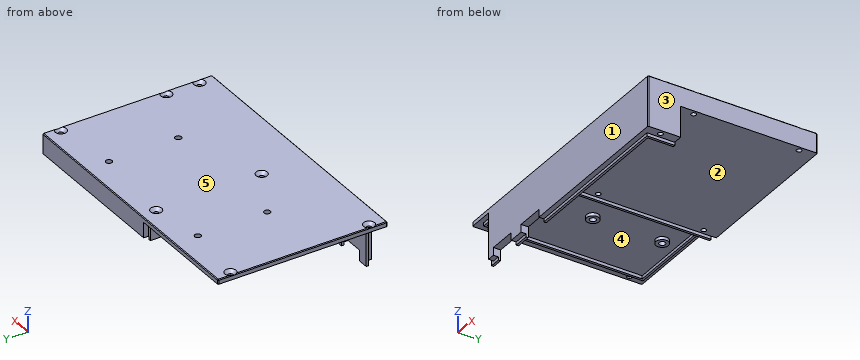
from build123d import *

# Parameters (mm, degrees)
ESQUISSE1_W             = 177.7
ESQUISSE1_H             = 110
BOSS_EXTRU_1_DEPTH      = 3
ESQUISSE2_W             = 102.6
ESQUISSE2_H             = 88.6
BOSS_EXTRU_2_DEPTH      = 10
BOSS_EXTRU_3_DEPTH      = 30
ESQUISSE4_W             = 6.1
ESQUISSE4_H             = 20
ENL_V_MAT_EXTRU_1_DEPTH = 0.2
ESQUISSE5_W             = 10
ESQUISSE5_H             = 3.2
ENL_V_MAT_EXTRU_2_DEPTH = 0.2
BOSS_EXTRU_4_DEPTH      = 2
BOSS_EXTRU_5_DEPTH      = 10
BOSS_EXTRU_6_DEPTH      = 30
ESQUISSE9_R             = 1.6
ENL_V_MAT_EXTRU_3_DEPTH = 212.901604524
CHANFREIN1_SIZE         = 2
CHANFREIN2_SIZE         = 0.5
ESQUISSE10_R            = 2
ENL_V_MAT_EXTRU_4_DEPTH = 5
ESQUISSE11_R            = 4
ESQUISSE11_R_2          = 2
BOSS_EXTRU_7_DEPTH      = 5
ESQUISSE13_W            = 18
ESQUISSE13_H            = 4.7
ENL_V_MAT_EXTRU_5_DEPTH = 7
ESQUISSE14_W            = 96.5
ESQUISSE14_H            = 0.5
BOSS_EXTRU_8_DEPTH      = 2


with BuildPart() as part:
    # Esquisse1 → Boss.-Extru.1 (new body)
    with BuildSketch(Plane.XY):
        with Locations((88.85, 55)):
            Rectangle(ESQUISSE1_W, ESQUISSE1_H)
    extrude(amount=BOSS_EXTRU_1_DEPTH)

    # Esquisse2 → Boss.-Extru.2 (add)
    with BuildSketch(Plane(origin=(0, 0, 0), x_dir=(-1, 0, 0), z_dir=(0, 0, -1))):
        with Locations((-126.4, 65.7)):
            Rectangle(ESQUISSE2_W, ESQUISSE2_H)
    extrude(amount=BOSS_EXTRU_2_DEPTH)

    # Esquisse3 → Boss.-Extru.3 (add)
    with BuildSketch(Plane(origin=(0, 0, 0), x_dir=(-1, 0, 0), z_dir=(0, 0, -1))):
        Polygon((-177.7, 21.4), (-171.6, 21.4), (-171.6, 3.2), (-16.2, 3.2), (-16.2, 0), (-177.7, 0), align=None)
    extrude(amount=BOSS_EXTRU_3_DEPTH)

    # Esquisse4 → Enlèv. mat.-Extru.1 (cut)
    with BuildSketch(Plane(origin=(0, 21.4, 0), x_dir=(1, 0, 0), z_dir=(0, 1, 0))):
        with Locations((174.65, 20)):
            Rectangle(ESQUISSE4_W, ESQUISSE4_H)
    extrude(amount=-ENL_V_MAT_EXTRU_1_DEPTH, mode=Mode.SUBTRACT)

    # Esquisse5 → Enlèv. mat.-Extru.2 (cut)
    with BuildSketch(Plane.ZY.offset(-75.1)):
        with Locations((-5, 108.4)):
            Rectangle(ESQUISSE5_W, ESQUISSE5_H)
    extrude(amount=-ENL_V_MAT_EXTRU_2_DEPTH, mode=Mode.SUBTRACT)

    # Esquisse6 → Boss.-Extru.4 (add)
    with BuildSketch(Plane(origin=(0, 0, 0), x_dir=(-1, 0, 0), z_dir=(0, 0, -1))):
        Polygon((-75.1, 106.8), (-6.1, 106.8), (-6.1, 3.2), (-171.6, 3.2), (-171.6, 21.4), (-75.1, 21.4), align=None)
        Polygon((-73.6, 105.3), (-7.6, 105.3), (-7.6, 4.7), (-170.1, 4.7), (-170.1, 19.9), (-73.6, 19.9), align=None, mode=Mode.SUBTRACT)
    extrude(amount=BOSS_EXTRU_4_DEPTH)

    # Esquisse7 → Boss.-Extru.5 (add)
    with BuildSketch(Plane(origin=(0, 0, -2), x_dir=(-1, 0, 0), z_dir=(0, 0, -1))):
        Polygon((-75.1, 106.8), (-73.6, 106.8), (-73.6, 19.4), (-171.6, 19.4), (-171.6, 21.4), (-75.1, 21.4), align=None)
    extrude(amount=BOSS_EXTRU_5_DEPTH)

    # Esquisse8 → Boss.-Extru.6 (add)
    with BuildSketch(Plane(origin=(0, 0, -2), x_dir=(-1, 0, 0), z_dir=(0, 0, -1))):
        Polygon((-14.2, 3.2), (-14.2, 4.7), (-170.1, 4.7), (-170.1, 21.4), (-171.6, 21.4), (-171.6, 3.2), align=None)
    extrude(amount=BOSS_EXTRU_6_DEPTH)

    # Esquisse9 → Enlèv. mat.-Extru.3 (cut, through all)
    with BuildSketch(Plane.XY.offset(3)):
        with Locations((3, 100)):
            Circle(ESQUISSE9_R)
        with Locations((3, 10)):
            Circle(ESQUISSE9_R)
        with Locations((174.7, 100)):
            Circle(ESQUISSE9_R)
        with Locations((174.7, 10)):
            Circle(ESQUISSE9_R)
        with Locations((78.2, 100)):
            Circle(ESQUISSE9_R)
        with Locations((78.2, 31.5)):
            Circle(ESQUISSE9_R)
        with Locations((174.7, 31.5)):
            Circle(ESQUISSE9_R)
    extrude(amount=-ENL_V_MAT_EXTRU_3_DEPTH, mode=Mode.SUBTRACT)

    # Chanfrein1
    # the kernel refuses this chamfer: 2 mm, written as the material it takes off along each edge
    with BuildSketch(Plane(origin=(78.2, 100, 3), x_dir=(1, 0, 0), z_dir=(0, -1, 0))) as chanfrein1_piece_1:
        Polygon((1.6 + CHANFREIN1_SIZE, 0), (1.6, -CHANFREIN1_SIZE), (1.6, 0), align=None)
    revolve(axis=Axis((78.2, 100, 3), (0, 0, 1)), mode=Mode.SUBTRACT)
    with BuildSketch(Plane(origin=(174.7, 10, 3), x_dir=(1, 0, 0), z_dir=(0, -1, 0))) as chanfrein1_piece_2:
        Polygon((1.6 + CHANFREIN1_SIZE, 0), (1.6, -CHANFREIN1_SIZE), (1.6, 0), align=None)
    revolve(axis=Axis((174.7, 10, 3), (0, 0, 1)), mode=Mode.SUBTRACT)
    with BuildSketch(Plane(origin=(174.7, 100, 3), x_dir=(1, 0, 0), z_dir=(0, -1, 0))) as chanfrein1_piece_3:
        Polygon((1.6 + CHANFREIN1_SIZE, 0), (1.6, -CHANFREIN1_SIZE), (1.6, 0), align=None)
    revolve(axis=Axis((174.7, 100, 3), (0, 0, 1)), mode=Mode.SUBTRACT)
    with BuildSketch(Plane(origin=(3, 10, 3), x_dir=(1, 0, 0), z_dir=(0, -1, 0))) as chanfrein1_piece_4:
        Polygon((1.6 + CHANFREIN1_SIZE, 0), (1.6, -CHANFREIN1_SIZE), (1.6, 0), align=None)
    revolve(axis=Axis((3, 10, 3), (0, 0, 1)), mode=Mode.SUBTRACT)
    with BuildSketch(Plane(origin=(78.2, 31.5, 3), x_dir=(1, 0, 0), z_dir=(0, -1, 0))) as chanfrein1_piece_5:
        Polygon((1.6 + CHANFREIN1_SIZE, 0), (1.6, -CHANFREIN1_SIZE), (1.6, 0), align=None)
    revolve(axis=Axis((78.2, 31.5, 3), (0, 0, 1)), mode=Mode.SUBTRACT)
    with BuildSketch(Plane(origin=(174.7, 31.5, 3), x_dir=(1, 0, 0), z_dir=(0, -1, 0))) as chanfrein1_piece_6:
        Polygon((1.6 + CHANFREIN1_SIZE, 0), (1.6, -CHANFREIN1_SIZE), (1.6, 0), align=None)
    revolve(axis=Axis((174.7, 31.5, 3), (0, 0, 1)), mode=Mode.SUBTRACT)
    with BuildSketch(Plane(origin=(3, 100, 3), x_dir=(1, 0, 0), z_dir=(0, -1, 0))) as chanfrein1_piece_7:
        Polygon((1.6 + CHANFREIN1_SIZE, 0), (1.6, -CHANFREIN1_SIZE), (1.6, 0), align=None)
    revolve(axis=Axis((3, 100, 3), (0, 0, 1)), mode=Mode.SUBTRACT)

    # Chanfrein2
    chanfrein2_edges = [part.edges().sort_by_distance(p)[0] for p in [
        (177.7, 65.75, 3),
        (177.7, 20.75, 3),
        (0, 4.005012563, 3),
        (177.7, 4.005012563, 3),
        (88.85, 0, 3),
        (0, 55, 3),
        (177.7, 105.994987437, 3),
        (0, 105.994987437, 3),
        (88.85, 110, 3),
        (0, 0, 1.5),
        (177.7, 0, -13.5),
        (0, 110, 1.5),
        (177.7, 110, -3.5),
    ]]
    chamfer(chanfrein2_edges, length=CHANFREIN2_SIZE)

    # Esquisse10 → Enlèv. mat.-Extru.4 (cut)
    with BuildSketch(Plane.XY.offset(3)):
        with Locations((43.85, 95)):
            Circle(ESQUISSE10_R)
        with Locations((43.85, 50)):
            Circle(ESQUISSE10_R)
        with Locations((133.85, 95)):
            Circle(ESQUISSE10_R)
        with Locations((133.85, 50)):
            Circle(ESQUISSE10_R)
    extrude(amount=-ENL_V_MAT_EXTRU_4_DEPTH, mode=Mode.SUBTRACT)

    # Esquisse11 → Boss.-Extru.7 (add)
    # profile 1 of 4: a face of its own
    with BuildSketch(Plane.XY.offset(3)):
        with Locations((43.85, 95)):
            Circle(ESQUISSE11_R)
        with Locations((43.85, 95)):
            Circle(ESQUISSE11_R_2, mode=Mode.SUBTRACT)
    # profile 2 of 4: a face of its own
    with BuildSketch(Plane.XY.offset(3)):
        with Locations((43.85, 50)):
            Circle(ESQUISSE11_R)
        with Locations((43.85, 50)):
            Circle(ESQUISSE11_R_2, mode=Mode.SUBTRACT)
    # profile 3 of 4: a face of its own
    with BuildSketch(Plane.XY.offset(3)):
        with Locations((133.85, 95)):
            Circle(ESQUISSE11_R)
        with Locations((133.85, 95)):
            Circle(ESQUISSE11_R_2, mode=Mode.SUBTRACT)
    # profile 4 of 4: a face of its own
    with BuildSketch(Plane.XY.offset(3)):
        with Locations((133.85, 50)):
            Circle(ESQUISSE11_R)
        with Locations((133.85, 50)):
            Circle(ESQUISSE11_R_2, mode=Mode.SUBTRACT)
    extrude(amount=-BOSS_EXTRU_7_DEPTH)

    # Esquisse13 → Enlèv. mat.-Extru.5 (cut)
    with BuildSketch(Plane(origin=(0, 0, -32), x_dir=(-1, 0, 0), z_dir=(0, 0, -1))):
        with Locations((-30.2, 2.35)):
            Rectangle(ESQUISSE13_W, ESQUISSE13_H)
        with Locations((-58.2, 2.35)):
            Rectangle(ESQUISSE13_W, ESQUISSE13_H)
    extrude(amount=-ENL_V_MAT_EXTRU_5_DEPTH, mode=Mode.SUBTRACT)

    # Esquisse14 → Boss.-Extru.8 (add)
    with BuildSketch(Plane.XY.offset(-2)):
        with Locations((121.85, 19.65)):
            Rectangle(ESQUISSE14_W, ESQUISSE14_H)
    extrude(amount=BOSS_EXTRU_8_DEPTH)


solid = part.part
Can you work these out from the model? Positions are in its coordinate system, mm. Face numbers are marked on the shaded views. A direction names the side the tool comes from. Round coordinates to 2 decimals unless told otherwise and drop trailing zeros. Write each loop counter-clockwise with the first axis right and the second up, starting at its lowest first coordinate (ties: lowest second). Pieces come first, ordered by that corner, then holes. Notation, with made-up numbers: M 26.5,-0.75 L 60.5,-0.75 A9 ccw 60.5,4.25 Z; hole C -20.75,56.5 d9. An arc over 180 degrees is marked long. Use a Markdown table: item, result.
Item 1: I want a section at A-A (z = -27). List the corners of the cut face in (x, y) for me.
Found:
| item | result |
|---|---|
| outline | M 14.2,3.2 L 16.2,3.2 L 16.2,0 L 21.2,0 L 21.2,4.7 L 14.2,4.7 Z; M 39.2,0 L 49.2,0 L 49.2,4.7 L 39.2,4.7 Z; M 67.2,0 L 177.2,0 L 177.7,0.5 L 177.7,21.2 L 171.6,21.2 L 171.6,21.4 L 170.1,21.4 L 170.1,4.7 L 67.2,4.7 Z; hole C 174.7,10 d3.2 |
Item 2: I want a section at B-B (x = 43.85). State how many separate pieces and enclosed holes the cut face has, and give its area (3 significant figures).
Found:
| item | result |
|---|---|
| separate pieces | 3 |
| enclosed holes | 0 |
| area | 469 mm2 |
Item 3: Which directions (+Z, -Z, +X, -X, +Y, -Y) give clear straight access to the entire face, cutting with the end or side of a thin tool? Please do the marked faces 1 and 2.
Found:
| item | result |
|---|---|
| face 1 | +Z, -Z, +X, -X, -Y |
| face 2 | -Z, +X, +Y |
Item 4: For pin 1 Ø4 at (x, y) = (26, 1.5) entering from -Z; pin 2 Ø1.6 at (x, y) = (18.5, 1.5) entering from -Z; pin 3 Ø3 at (x, z) = (174, -23) entering from +Y; pin 4 Ø2.5 at (x, y) = (43.5, 95) entering from -Z, each with a flat end and sliding along its axis, tell me the tip position at first contact or that it passes through.
Found:
| item | result |
|---|---|
| pin 1 | stops at z = -25 |
| pin 2 | stops at z = -30 |
| pin 3 | stops at y = 21.2 |
| pin 4 | passes through |
Item 5: If I drill on line 1 along Y through (x, z) = (43.85, 2); line 2 along Y through (x, z) = (3, 0.35); line 3 along Y through (x, z) = (102.5, -9.5), over which ranges is the centre line in solid material (lowest first)? Write a range as [from, to].
Found:
| item | result |
|---|---|
| line 1 | y = [0, 48], [52, 93], [97, 110] |
| line 2 | y = [0, 8.4], [11.6, 98.4], [101.6, 110] |
| line 3 | y = [0, 4.7], [19.4, 110] |
Item 6: I want a section at D-D (x = 146). List the corners of the cut face in (y, z) for me, and give its area (3 significant figures).
Found:
| item | result |
|---|---|
| outline | M 0,-30 L 3.2,-30 L 3.2,-32 L 4.7,-32 L 4.7,0 L 19.4,0 L 19.4,-12 L 21.4,-12 L 21.4,-10 L 110,-10 L 110,2.5 L 109.5,3 L 0.5,3 L 0,2.5 Z |
| area | 1,380 mm2 |
Item 7: I want a section at C-C (y = 69.5). List the corners of the cut face in (x, z) for me, and give its area (3 significant figures).
Found:
| item | result |
|---|---|
| outline | M 0,0 L 6.1,0 L 6.1,-2 L 7.6,-2 L 7.6,0 L 73.6,0 L 73.6,-12 L 75.1,-12 L 75.1,-10 L 177.7,-10 L 177.7,2.5 L 177.2,3 L 0.5,3 L 0,2.5 Z |
| area | 1,580 mm2 |
Item 8: We'd pull the mould along X, two halves only. Please class the marked faces 3, 4 and 5: released by +X, released by -X, zero draft, split by the parting line, or undercut.
Found:
| item | result |
|---|---|
| face 3 | released by +X |
| face 4 | undercut |
| face 5 | zero draft |
